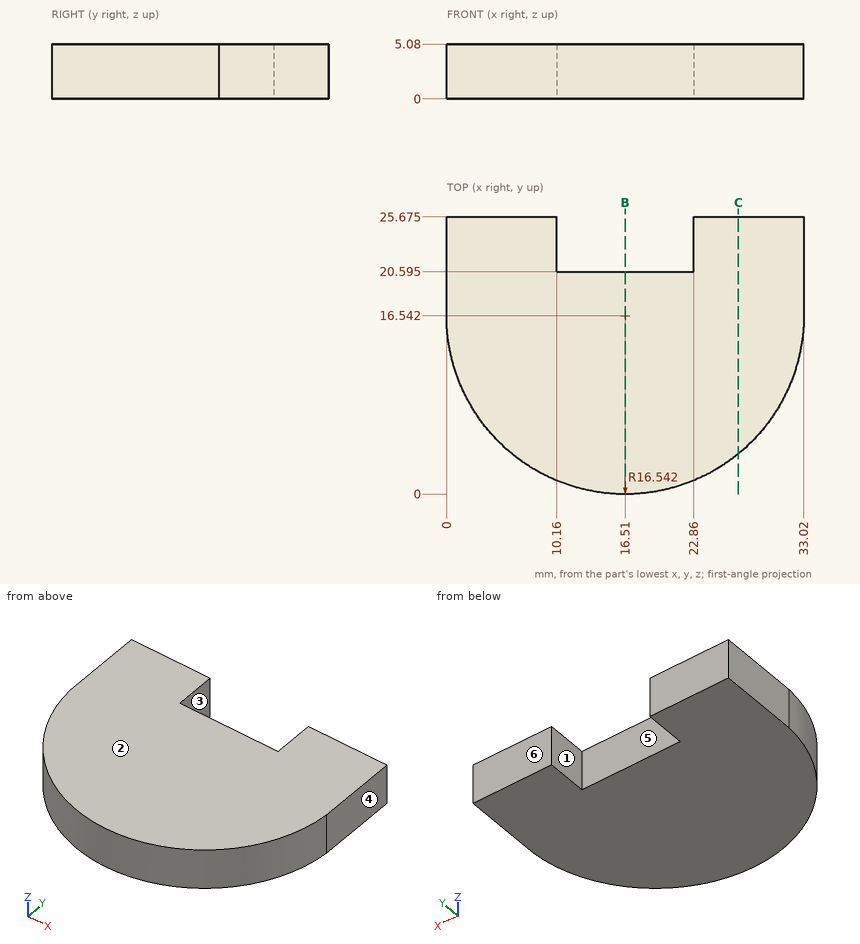
Print and shaded views of the part. All mm, measured from the part's lowest x, y and z. A direction names the side the tool comes from. Round coordinates to 2 decimals unless told otherwise and drop trailing zeros. Order: outer loops, then holes, each group sorted by start corner. A loop starts at its lowest first (then second) coordinate and runs counter-clockwise, first axis right, second up.
Q1. Two-plate mould, pull along X, no slides. Class the marked faces 3, 4, 5 and 6: pulls with the +X half, pulls with the -X half, needs draft (parallel to the pull), parting line crosses it, or undercut.
Q2. Which spindle directions (+Z, -Z, +X, -X, +Y, -Y) get a long thin tool onto all of the face, cutting with end or side? Do the marked faces 1 and 2. Say none if no direction does.
Q3. Drop a flat-ended pin along its axis: pin 1 (3 mm diameter, centred on y = 5, z = 1.5, fed in from -X) (1 decimal). Give the stop position or say it passes through.
Q4. Slice it at B-B (x = 16.51). Write the cut outline in (y, z) (1 decimal), and give its area (3 significant figures).
Q5. Slice it at C-C (x = 27). Write the cut outline in (y, z) (1 decimal).
Q6. Wall check: L1, parallel to X at y = 22, z = 3.35; L2, parallel to Y at x = 16.5, z = 3.55 (1 decimal); L3, parallel to X at y = 15.5, z = 2.7. Give the ranges that are in metal, low to high.
Results below:
1. face 3: undercut
1. face 4: pulls with the +X half
1. face 5: undercut
1. face 6: needs draft
2. face 1: +Z, -Z, +Y
2. face 2: +Z, +X, -X, +Y, -Y
3. pin 1: stops at x = 3.4
4. outline: (0, 0) - (20.6, 0) - (20.6, 5.1) - (0, 5.1) - close
4. area: 105 mm2
5. outline: (3.8, 0) - (25.7, 0) - (25.7, 5.1) - (3.8, 5.1) - close
6. L1: x = 0 to 10.16, 22.86 to 33.02
6. L2: y = 0 to 20.6
6. L3: x = 0 to 33.02
